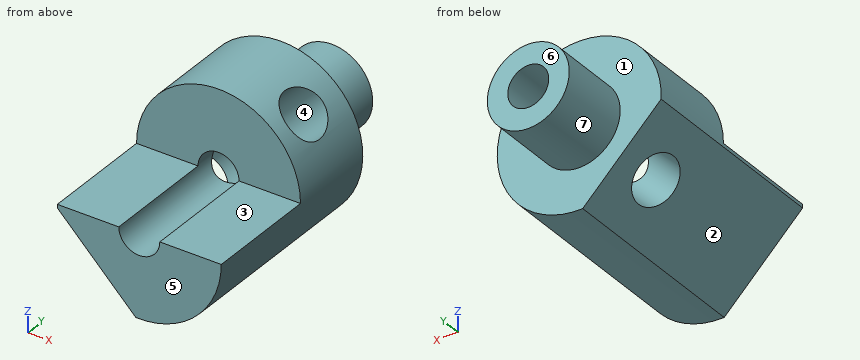
from build123d import *

# Parameters (mm, degrees)
CUT_EXTRUDE_1_DEPTH             = 7
CUT_EXTRUDE_2_DEPTH             = 18
SKETCH_5_R                      = 1.5
CUT_EXTRUDE_3_DEPTH             = 4.388378183
CUT_EXTRUDE_3_DIRECTION_2_REACH = 12.754


with BuildPart() as part:
    # Эскиз1 → Повернуть1 (revolve)
    with BuildSketch(Plane(origin=(0, 0, 0), x_dir=(0, 0, -1), z_dir=(1, 0, 0))):
        Polygon((2.5, -4.5), (2.5, 0), (1.25, 0), (1.25, -17), (5, -17), (5, -4.5), align=None)
    revolve(axis=Axis((0, 0, 0), (0, -1, 0)))

    # Эскиз2 → Вырез-Вытянуть1 (cut)
    with BuildSketch(Plane.XZ.offset(17)):
        Polygon((-37.360679775, 0), (-5, 0), (5, 0), (37.360679775, 0), (37.360679775, 64.72135955), (-37.360679775, 64.72135955), align=None)
    extrude(amount=-CUT_EXTRUDE_1_DEPTH, mode=Mode.SUBTRACT)

    # Эскиз3 → Вырез-Вытянуть2 (cut, through all)
    with BuildSketch(Plane.XZ.offset(17)):
        with BuildLine():
            Line((-0.212632943, -4.995476677), (-4.995476677, -0.212632943))
            ThreePointArc((-4.995476677, -0.212632943), (-3.535533906, -3.535533906), (-0.212632943, -4.995476677))
        make_face()
    extrude(amount=-CUT_EXTRUDE_2_DEPTH, mode=Mode.SUBTRACT)

    # Эскиз5 → Вырез-Вытянуть3 (cut)
    with BuildSketch(Plane(origin=(-7.70810962, 0, 2.5), x_dir=(0.707106781, 0, -0.707106781), z_dir=(0.707106781, 0, 0.707106781))):
        with Locations((7.218223535, -7.5)):
            Circle(SKETCH_5_R)
    extrude(amount=-CUT_EXTRUDE_3_DEPTH, mode=Mode.SUBTRACT)

    # Эскиз5 → Вырез-Вытянуть3 direction 2 (cut, up to next)
    with BuildSketch(Plane(origin=(-7.70810962, 0, 2.5), x_dir=(0.707106781, 0, -0.707106781), z_dir=(0.707106781, 0, 0.707106781)), mode=Mode.PRIVATE) as cut_extrude_3_direction_2_sk1:
        with Locations((7.218223535, -7.5)):
            Circle(SKETCH_5_R)
    cut_extrude_3_direction_2_tool1 = extrude(cut_extrude_3_direction_2_sk1.sketch, amount=CUT_EXTRUDE_3_DIRECTION_2_REACH, mode=Mode.PRIVATE) & part.part
    add(cut_extrude_3_direction_2_tool1.solids().sort_by_distance((-2.604055, -7.5, -2.604055))[0], mode=Mode.SUBTRACT)


solid = part.part
Build history of the part. All positions in model axes, mm. Face numbers are marked on the shaded views. A direction names the side the tool comes from. Coordinates: 2 decimals unless noted, no trailing zeros. Order: outer loops, then holes, each group sorted by start corner. A loop starts at its lowest first (then second) coordinate and runs counter-clockwise, first axis right, second up. Notation, with made-up numbers: (-15, 79) - (9, 79) arc R14 ccw to (9, 93) - close; hole circle Ø11 at (-5, -36). An arc over 180 degrees is marked (long way). Put each result on its own line as item: value.
1. Drop flat-ended pins along their axis: P1, Ø3, axis at x = -3, y = -14, coming from the +Z side; P2, Ø4, axis at x = 0.5, z = 3.5, coming from the -Y side; P3, Ø4, axis at y = -6, z = 3.5, coming from the -X side; P4, Ø2, axis at x = 0, z = 0, coming from the -Y side. Give the stop position or say it passes through.
Answer sheet:
P1: stops at z = 0
P2: stops at y = -10
P3: stops at x = -4.77
P4: passes through
2. Saw through at B-B (y = -14). Write the cut outline in (x, z).
Answer sheet:
outline: (-5, -0.21) - (-0.21, -5) arc R5 ccw to (5, 0) - (1.25, 0) arc R1.25 cw to (-1.25, 0) - (-5, 0) arc R5 ccw to start
3. Probe line 1 along X through (y, z) = (-2, 0); line 2 along Y through (x, z) = (-1.25, 2.25); line 3 along Z through (x, y) = (-0.75, -3.5). List the from-to ranges inside material, lowest first. Write a range as [from, to].
Answer sheet:
line 1: x = [-2.5, -1.25], [1.25, 2.5]
line 2: y = [-10, -4.5]
line 3: z = [-2.38, -1], [1, 2.38]
4. Pull direction Y, two halves, no side cores. Call the marked faces 4, 5, 6 and 7: pulls with the +Y half, pulls with the -Y half, needs draft (parallel to the pull), parting line crosses it, or undercut.
Answer sheet:
face 4: undercut
face 5: pulls with the -Y half
face 6: pulls with the +Y half
face 7: needs draft
5. Saw through at A-A (y = -5.5). Write the cut outline in (x, z), and give its area (3 significant figures).
Answer sheet:
outline: (-5, -0.21) - (-0.21, -5) arc R5 ccw (long way) to start; hole circle Ø2.5 at (0, 0)
area: 67.5 mm^2
6. Tool access for the marked faces 1, 2 and 3: list every direction of +Z, -Z, +X, -X, +Y, -Y with a clear straight run to the whole face (end or side of a thin tool).
Answer sheet:
face 1: +Y
face 2: -Z, -X, +Y, -Y
face 3: +Z, +X, -X, -Y
7. Saw through at C-C (x = -4.5). Write the cut outline in (y, z), and give its area (3 significant figures).
Answer sheet:
outline: (-17, -0.71) - (-4.5, -0.71) - (-4.5, 2.18) - (-10, 2.18) - (-10, 0) - (-17, 0) - close
area: 20.8 mm^2
